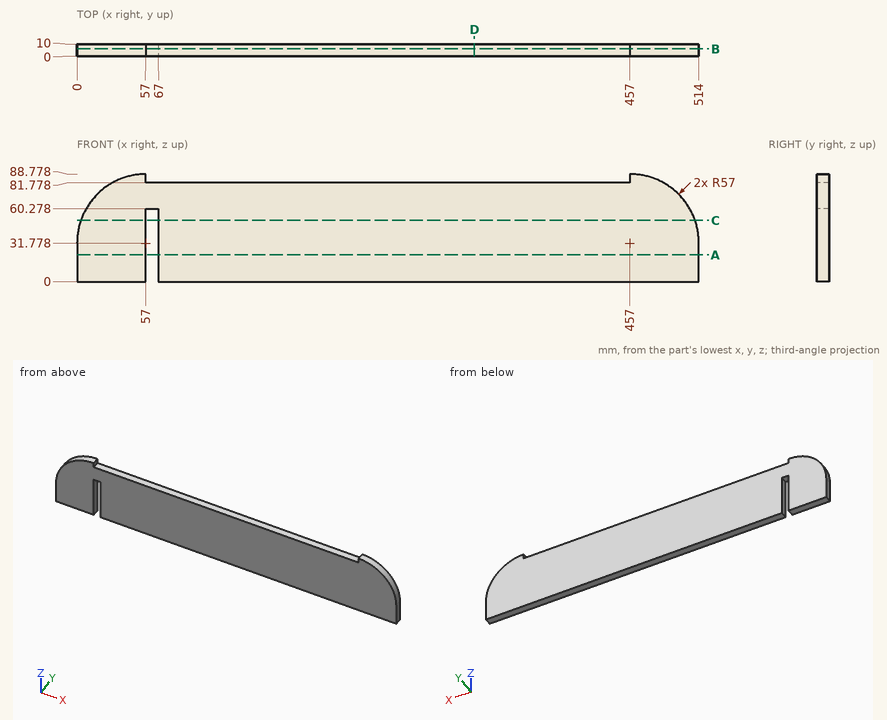
Source: three-view drawing plus pictorial views. Frame: mm from the lowest corner of the part. Give positions to 0.01 mm unless a question says otherwise; leave off trailing zeros. Order: outer loops, then holes, each group sorted by start corner. A loop starts at its lowest first (then second) coordinate and runs counter-clockwise, first axis right, second up.
1. Section B-B on y = 6. Return the cut outline in (x, z), and give its area (3 significant figures).
Derived:
outline: (0, 0) - (57, 0) - (57, 60.28) - (67, 60.28) - (67, 0) - (514, 0) - (514, 31.78) arc R57 ccw to (457, 88.78) - (457, 81.78) - (57, 81.78) - (57, 88.78) arc R57 ccw to (0, 31.78) - close
area: 40,800 mm2
2. Section D-D on x = 328.5. Return the cut outline in (y, z), and give its area (3 significant figures).
Derived:
outline: (0, 0) - (10, 0) - (10, 81.78) - (0, 81.78) - close
area: 818 mm2
3. Material intervals for L1, parallel to X at y = 8.5, z = 31.5; L2, parallel to Z at x = 281, y = 9.75; L3, parallel to X at y = 3, z = 41, sorted ascending.
Derived:
L1: x = 0 to 57, 67 to 514
L2: z = 0 to 81.78
L3: x = 0.75 to 57, 67 to 513.25
4. Section A-A on z = 22. Return the cut outline in (x, y).
Derived:
outline: (0, 0) - (57, 0) - (57, 10) - (0, 10) - close; (67, 0) - (514, 0) - (514, 10) - (67, 10) - close
5. Section C-C on z = 50.5. Return the cut outline in (x, y).
Derived:
outline: (3.16, 0) - (57, 0) - (57, 10) - (3.16, 10) - close; (67, 0) - (510.84, 0) - (510.84, 10) - (67, 10) - close
6. Pin query (flat end, axial travel): pin 1 (3 mm diameter, centred on x = 257, y = 5, fed in from +Z); pin 2 (3.5 mm diameter, centred on y = 3.5, z = 86, fed in from -X) (1 decimal); pin 3 (4 mm diameter, centred on y = 7, z = 69, fed in from +X) (1 decimal). Return the tip coordinate at first contact, or that it passes through.
Derived:
pin 1: stops at z = 81.78
pin 2: stops at x = 34.7
pin 3: stops at x = 501.8
